Autodesk Inventor part; units mm, degrees
ref_plane "YZ Plane" through (0, 0, 0) normal (1, 0, 0) x (0, 1, 0)
ref_plane "XZ Plane" through (0, 0, 0) normal (0, 1, 0) x (-1, 0, 0)
ref_plane "XY Plane" through (0, 0, 0) normal (0, 0, 1) x (1, 0, 0)
sketch "Sketch1" plane through (0, 0, 0) normal (0, 1, 0) x (-1, 0, 0)
  line L0 (0, 0) -> (-48, 0)
  line L1 (-48, 0) -> (-48, -43)
  line L2 (-48, -43) -> (0, -43)
  line L3 (0, -43) -> (0, 0)
  circle A0 centre (-24, -27.5) radius 1.95
  circle A1 centre (-24, -12.5) radius 1.95
  circle A2 centre (-8, -5.5) radius 1.95
  circle A3 centre (-40, -5.5) radius 1.95
  circle A4 centre (-40, -37.5) radius 1.95
  circle A5 centre (-8, -37.5) radius 1.95
  point P0 (-24, -43)
  dimension "d0" = 48
  dimension "d1" = 43
  dimension "d2" = 3.9
  dimension "d3" = 3.9
  dimension "d4" = 15
  dimension "d5" = 12.5
  dimension "d6" = 3.9
  dimension "d7" = 3.9
  dimension "d8" = 3.9
  dimension "d9" = 3.9
  dimension "d10" = 32
  dimension "d11" = 8
  dimension "d12" = 5.5
  dimension "d13" = 5.5
extrude "Extrusion1" add sketch "Sketch1" along normal blind 15
sketch "Sketch2" plane through (0, 15, 0) normal (0, 1, 0) x (1, 0, 0)
  line L0 (14, 49.9518) -> (34, 49.9518)
  line L1 (34, 49.9518) -> (34, -4.9916)
  line L2 (34, -4.9916) -> (14, -4.9916)
  line L3 (14, -4.9916) -> (14, 49.9518)
  line L4 (48, 43) -> (0, 43)
  point P0 (0, 0)
  point P1 (24, 49.9518)
  point P2 (24, 43)
  dimension "d16" = 20
extrude "Extrusion2" cut sketch "Sketch2" against normal blind 5
sketch "Sketch3" plane through (48, 0, -43) normal (0, 0, -1) x (-1, 0, 0)
  circle A0 centre (16, 5.5) radius 1.95
  circle A1 centre (24, 5.5) radius 1.95
  circle A2 centre (32, 5.5) radius 1.95
  line L0 (34, 10) -> (14, 10)
  line L1 (0, 0) -> (48, 0)
  circle A3 centre (8, 5.5) radius 1.95
  circle A4 centre (40, 5.5) radius 1.95
  circle A5 centre (0, 5.5) radius 1.95
  circle A6 centre (48, 5.5) radius 1.95
  point P0 (24, 10)
  dimension "d19" = 3.9
  dimension "d20" = 3.9
  dimension "d21" = 3.9
  dimension "d22" = 8
  dimension "d23" = 8
  dimension "d24" = 5.5
  dimension "d25" = 3.9
  dimension "d26" = 3.9
  dimension "d27" = 8
  dimension "d28" = 8
  dimension "d29" = 3.9
  dimension "d30" = 3.9
  dimension "d31" = 8
  dimension "d32" = 8
extrude "Extrusion3" cut sketch "Sketch3" against normal through all contours A0 | A2 | A3 | A4 | A5 | A6
sketch "Sketch4" plane through (0, 0, 0) normal (0, -1, 0) x (1, 0, 0)
  circle A0 centre (16, -5.5) radius 3.75
  circle A1 centre (16, -37.5) radius 3.75
  circle A2 centre (32, -37.5) radius 3.75
  circle A3 centre (32, -5.5) radius 3.75
  line L0 (0, 0) -> (48, 0)
  circle A4 centre (40, -5.5) radius 1.95
  dimension "d35" = 7.5
  dimension "d36" = 7.5
  dimension "d37" = 7.5
  dimension "d38" = 7.5
  dimension "d39" = 16
  dimension "d40" = 5.5
  dimension "d41" = 8
  dimension "d42" = 32
extrude "Extrusion4" cut sketch "Sketch4" against normal blind 5 contours A0 | A1 | A2 | A3
fillet "Fillet1" radius 1 11 edges at (14, 15, -21.5) (34, 15, -21.5) (0, 15, -21.5) (48, 15, -21.5) (7, 15, -43) (41, 15, -43) (7, 15, 0) (41, 15, 0) (34, 12.5, -43) (14, 12.5, -43) (24, 10, -43)
sketch "Sketch5" plane through (0, 15, 0) normal (0, 1, 0) x (1, 0, 0)
  circle A0 centre (8, 5.5) radius 3.65
  circle A1 centre (40, 5.5) radius 3.65
  circle A2 centre (8, 37.5) radius 3.65
  circle A3 centre (40, 37.5) radius 3.65
  circle A4 centre (40, 37.5) radius 1.95
  circle A5 centre (40, 5.5) radius 1.95
  circle A6 centre (8, 37.5) radius 1.95
  point P0 (0, 0)
  dimension "d46" = 7.3
  dimension "d47" = 7.3
  dimension "d48" = 7.3
  dimension "d49" = 7.3
extrude "Extrusion5" cut sketch "Sketch5" against normal blind 4
sketch "Sketch6" plane through (0, 0, 0) normal (0, -1, 0) x (1, 0, 0)
  line L0 (21.8927, -23.85) -> (26.1073, -23.85)
  line L1 (26.1073, -23.85) -> (28.2147, -27.5)
  line L2 (28.2147, -27.5) -> (26.1073, -31.15)
  line L3 (26.1073, -31.15) -> (21.8927, -31.15)
  line L4 (21.8927, -31.15) -> (19.7853, -27.5)
  line L5 (19.7853, -27.5) -> (21.8927, -23.85)
  line L6 (48, -43) -> (0, -43)
  line L7 (48, 0) -> (48, -43)
  line L8 (0, 0) -> (48, 0)
  line L9 (26.1073, -16.15) -> (21.8927, -16.15)
  line L10 (21.8927, -16.15) -> (19.7853, -12.5)
  line L11 (19.7853, -12.5) -> (21.8927, -8.85)
  line L12 (21.8927, -8.85) -> (26.1073, -8.85)
  line L13 (26.1073, -8.85) -> (28.2147, -12.5)
  line L14 (28.2147, -12.5) -> (26.1073, -16.15)
  point P0 (24, -27.5)
  point P1 (24, -12.5)
  dimension "d52" = 7.3
  dimension "d53" = 24
  dimension "d55" = 27.5
  dimension "d56" = 7.3
  dimension "d57" = 12.5
  dimension "d58" = 24
extrude "Extrusion6" cut sketch "Sketch6" against normal blind 5
sketch "Sketch7" plane through (0, 15, 0) normal (0, 1, 0) x (1, 0, 0)
  line L0 (-2.812, 43.9982) -> (53.4288, 43.9982)
  line L1 (53.4288, 43.9982) -> (53.4288, -3.3264)
  line L2 (53.4288, -3.3264) -> (-2.812, -3.3264)
  line L3 (-2.812, -3.3264) -> (-2.812, 43.9982)
  point P0 (0, 0)
extrude "Extrusion7" cut sketch "Sketch7" against normal blind 2
fillet "Fillet2" radius 1 10 edges at (13.7071, 13, -42.7071) (6.5, 13, -43) (14, 13, -21) (34.2929, 13, -42.7071) (41.5, 13, -43) (34, 13, -21) (41, 13, 0) (48, 13, -21.5) (0, 13, -21.5) (7, 13, 0)
properties part number "slidesmount"
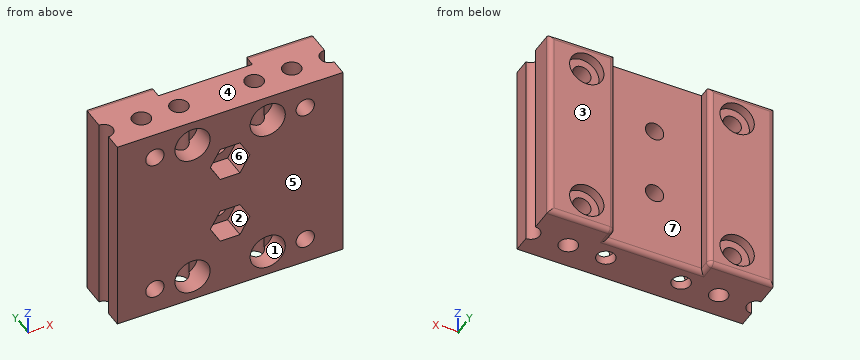
Could you check a few things on this model? Use its own coordinates, in mm. Face numbers are marked on the shaded views. A direction names the side the tool comes from. Round coordinates to 2 decimals unless told otherwise and drop trailing zeros. Loops run counter-clockwise (first coordinate to the right, second up) from the corner with the lowest first, then second, coordinate; pieces in that order, holes last. Notation, with made-up numbers: M 52.5,35.25 L 71.5,35.25 A20 cw 71.5,69.25 Z; hole C -11.75,47 d3. An arc over 180 degrees is marked long. Write item = value, one per line.
1. I want a section at B-B, the plane y = 2. Count the separate pieces of the cut face and the enclosed holes in it, and give its area (3 significant figures).
Results below:
separate_pieces = 1
enclosed_holes = 10
area = 1,750 mm²
2. I want a section at A-A, the plane z = -28.5. Write out the boundary of the cut face in (x, y).
Results below:
outline = M 0,0 L 20.36,0 L 20.36,5 L 22.33,5 L 22.33,10 L 14,10 L 14,12 A1 ccw 13,13 L 1,13 A1 ccw 0,12 L 0,7.45 A1.95 cw 0,3.55 Z; M 25.67,5 L 27.64,5 L 27.64,0 L 48,0 L 48,3.55 A1.95 cw 48,7.45 L 48,12 A1 ccw 47,13 L 35,13 A1 ccw 34,12 L 34,10 L 25.67,10 Z; hole C 8,5.5 d3.9; hole C 16,5.5 d3.9; hole C 32,5.5 d3.9; hole C 40,5.5 d3.9
3. Will these pins go through, and if not, where does the flat tip stop? P1, Ø5, axis at x = 24, z = -12.5, coming from the -Y side; P2, Ø4.5, axis at x = 8, z = -37.5, coming from the -Y side; P3, Ø2, axis at x = 38.5, z = -38, coming from the +Y side.
Results below:
P1 = 5
P2 = 0
P3 = 11
4. I want a section at D-D, the plane x = 32. Write out the boundary of the cut face in (y, z), and give its area (3 significant figures).
Results below:
outline = M 0,-43 L 3.55,-43 L 3.55,-41.25 L 0,-41.25 Z; M 0,-33.75 L 3.55,-33.75 L 3.55,-9.25 L 0,-9.25 Z; M 0,-1.75 L 3.55,-1.75 L 3.55,0 L 0,0 Z; M 7.45,-43 L 9,-43 A1 ccw 10,-42 L 10,0 L 7.45,0 Z
area = 209 mm²
5. Thinking about a two-plate mould opening in Z: for the marked faces 1, 2, 3 and 4, which applies, +Z half, -Z half, draft (parallel to the pull), parting line (faces both ways), or undercut?
Results below:
face_1 = undercut
face_2 = undercut
face_3 = draft
face_4 = +Z half
6. I need wall thicknesses on probe 1 along X at (y, z) = (9.85, -37.5); probe 2 along Z at (x, y) = (40, 9.35); probe 3 along X at (y, z) = (1.6, -37.5). Which ranges of each line are inside material? Lowest first, please.
Results below:
probe_1 = 0 to 6.05, 9.95 to 38.05, 41.95 to 48
probe_2 = -43 to -39.45, -35.55 to -7.45, -3.55 to 0
probe_3 = 0 to 6.05, 9.95 to 12.25, 19.75 to 28.25, 35.75 to 38.05, 41.95 to 48
7. Which directions (+Z, -Z, +X, -X, +Y, -Y) give clear straight access to the entire face, cutting with the end or side of a thin tool? Please do the marked faces 5, 6 and 7.
Results below:
face_5 = +Z, -Z, +X, -X, -Y
face_6 = -Y
face_7 = +Z, -Z, +Y
